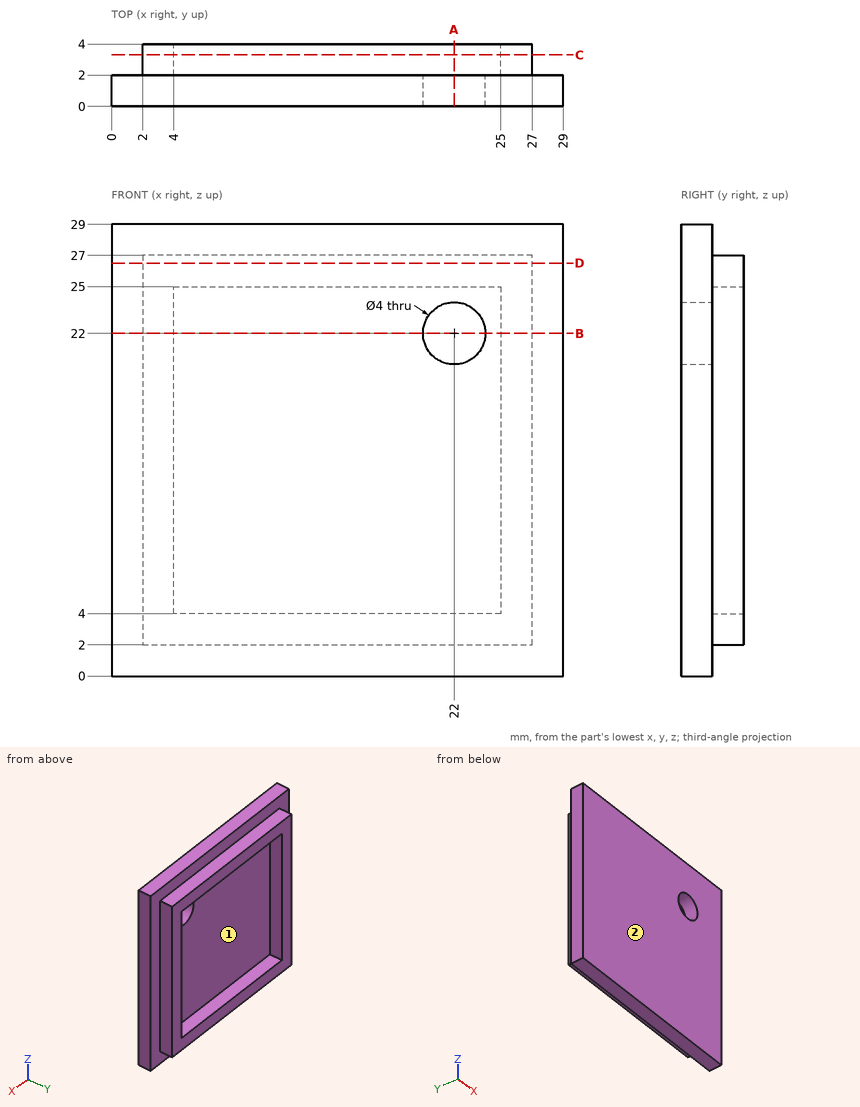
Here's the drawing with two shaded views (mm, measured from the low corner). I have some questions. Give positions to 0.01 mm unless a question says otherwise; leave off trailing zeros. Loops run counter-clockwise (first coordinate to the right, second up) from the corner with the lowest first, then second, coordinate; pieces in that order, holes last. Notation, with made-up numbers: (73.25, 43) - (79.25, 43) arc R18 cw to (79.25, 71) - close; hole circle Ø1 at (22, 16). An arc over 180 degrees is marked (long way). One line per item, written item: value.
(1) If we mould it in two halves opening along X, with no side actions, what happens to the marked faces 1 and 2? For each: released by +X, released by -X, zero draft, split by the parting line, or undercut.
Verdict:
face 1: undercut
face 2: zero draft
(2) If we section it at A-A, the plane x = 22: List the corners of the cut face in (y, z) for me.
Verdict:
outline: (0, 0) - (2, 0) - (2, 2) - (4, 2) - (4, 4) - (2, 4) - (2, 20) - (0, 20) - close; (0, 24) - (2, 24) - (2, 25) - (4, 25) - (4, 27) - (2, 27) - (2, 29) - (0, 29) - close
(3) If we section it at C-C, the plane y = 3.3: List the corners of the cut face in (x, z) for me.
Verdict:
outline: (2, 2) - (27, 2) - (27, 27) - (2, 27) - close; hole (4, 4) - (25, 4) - (25, 25) - (4, 25) - close
(4) I need wall thicknesses on line 1 along X through (y, z) = (1.55, 22); line 2 along X through (y, z) = (2.4, 11). Which ranges of each line are inside material? Lowest first, please.
Verdict:
line 1: 0 to 20, 24 to 29
line 2: 2 to 4, 25 to 27
(5) If we section it at D-D, the plane z = 26.5: List the corners of the cut face in (x, y) for me.
Verdict:
outline: (0, 0) - (29, 0) - (29, 2) - (27, 2) - (27, 4) - (2, 4) - (2, 2) - (0, 2) - close
(6) I'm going to push flat-ended pins straight in: pin 1 (6 mm diameter, centred on x = 3, z = 13.5, fed in from -Y); pin 2 (1.6 mm diameter, centred on x = 11.5, y = 3, fed in from -Z); pin 3 (17 mm diameter, centred on x = 14.5, z = 13.5, fed in from +Y); pin 4 (1.6 mm diameter, centred on x = 19, y = 3, fed in from +Z). Where does each tip first touch, or does it pass through?
Verdict:
pin 1: y = 0
pin 2: z = 2
pin 3: y = 2
pin 4: z = 27
(7) If we section it at B-B, the plane z = 22: List the corners of the cut face in (x, y) for me.
Verdict:
outline: (0, 0) - (20, 0) - (20, 2) - (4, 2) - (4, 4) - (2, 4) - (2, 2) - (0, 2) - close; (24, 0) - (29, 0) - (29, 2) - (27, 2) - (27, 4) - (25, 4) - (25, 2) - (24, 2) - close
